```python
from build123d import *

# Parameters (mm, degrees)
SKETCH_R           = 23
PAD_DEPTH          = 5
SKETCH001_R        = 2.7
POCKET_DEPTH       = 5
SKETCH002_W        = 5
SKETCH002_H        = 5
PAD001_DEPTH       = 100
POLARPATTERN_COUNT = 4
SKETCH003_R        = 23
PAD002_DEPTH       = 5


with BuildPart() as part:
    # Sketch → Pad (new body)
    with BuildSketch(Plane.XY):
        Circle(SKETCH_R)
    extrude(amount=PAD_DEPTH)

    # Sketch001 → Pocket (cut)
    with BuildSketch(Plane.XY):
        Circle(SKETCH001_R)
    extrude(amount=POCKET_DEPTH, mode=Mode.SUBTRACT)

    # Sketch002 → Pad001 (join)
    with BuildSketch(Plane.XY.offset(5)):
        with Locations((19.5, 0)):
            Rectangle(SKETCH002_W, SKETCH002_H)
    pad001 = extrude(amount=PAD001_DEPTH)

    # PolarPattern: Pad001 ×4 about axis
    polarpattern_axis = Axis((0, 0, 0), (0, 0, 1))
    for i in range(1, POLARPATTERN_COUNT):
        add(pad001.rotate(polarpattern_axis, i * 360 / POLARPATTERN_COUNT))

    # Sketch003 → Pad002 (join)
    with BuildSketch(Plane.XY.offset(105)):
        Circle(SKETCH003_R)
    extrude(amount=PAD002_DEPTH)


solid = part.part
```
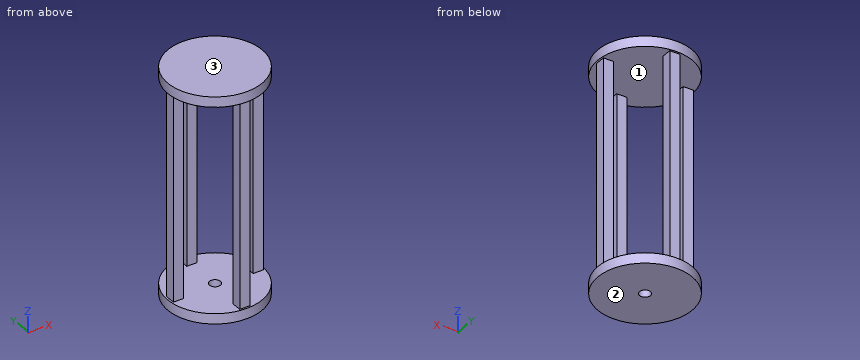
CAD build for the part. Positions are in the model's coordinates, mm. Face numbers are marked on the shaded views. Coordinates: 2 decimals unless noted, no trailing zeros. Order: outer loops, then holes, each group sorted by start corner. A loop starts at its lowest first (then second) coordinate and runs counter-clockwise, first axis right, second up.
(1) Drill centre lines: L1, parallel to Z at x = -20, y = 4; L2, parallel to Y at x = 0, z = 1; L3, parallel to Y at x = -0.5, z = 77.5. Where is each one in solid material? Low to high.
Solution:
L1: z = 0 to 5, 105 to 110
L2: y = -23 to -2.7, 2.7 to 23
L3: y = -22 to -17, 17 to 22
(2) Saw through at A-A, the plane y = -12. Write the cut outline in (x, z), and give its area (3 significant figures).
Solution:
outline: (-19.62, 0) - (19.62, 0) - (19.62, 5) - (-19.62, 5) - close; (-19.62, 105) - (19.62, 105) - (19.62, 110) - (-19.62, 110) - close
area: 392 mm2
(3) Mould opens along Z. For the marked faces 1, 2 and 3 say: released by +Z, released by -Z, zero draft, split by the parting line, or undercut.
Solution:
face 1: undercut
face 2: released by -Z
face 3: released by +Z
(4) Pin check, flat tips, straight feed: pin 1 Ø4 at (x, z) = (19.5, 67) entering from -Y; pin 2 Ø5.5 at (y, z) = (-19, 60) entering from +X; pin 3 Ø5 at (y, z) = (0, 32) entering from -X. Stop position of each tip, or through.
Solution:
pin 1: stops at y = -2.5
pin 2: stops at x = 2.5
pin 3: stops at x = -22
(5) Saw through at B-B, the plane z = 103.5. Write the cut outline in (x, y), and give its area (3 significant figures).
Solution:
outline: (-22, -2.5) - (-17, -2.5) - (-17, 2.5) - (-22, 2.5) - close; (-2.5, -22) - (2.5, -22) - (2.5, -17) - (-2.5, -17) - close; (-2.5, 17) - (2.5, 17) - (2.5, 22) - (-2.5, 22) - close; (17, -2.5) - (22, -2.5) - (22, 2.5) - (17, 2.5) - close
area: 100 mm2
(6) Saw through at C-C, the plane x = 0. Write the cut outline in (y, z), and give its area (3 significant figures).
Solution:
outline: (-23, 0) - (-2.7, 0) - (-2.7, 5) - (-17, 5) - (-17, 105) - (17, 105) - (17, 5) - (2.7, 5) - (2.7, 0) - (23, 0) - (23, 5) - (22, 5) - (22, 105) - (23, 105) - (23, 110) - (-23, 110) - (-23, 105) - (-22, 105) - (-22, 5) - (-23, 5) - close
area: 1,430 mm2
